For this review, take the finished solid that the model builds, in its own axes (mm). A direction names the side the tool comes from. Give positions to 0.01 mm unless a question says otherwise; leave off trailing zeros. Order: outer loops, then holes, each group sorted by start corner. A loop starts at its lowest first (then second) coordinate and runs counter-clockwise, first axis right, second up. Notation, with made-up numbers: (43.5, 28) - (58.5, 28) arc R30 cw to (58.5, 58) - close; hole circle Ø3 at (45.5, 65.5). An arc over 180 degrees is marked (long way). One line per item, written item: value.
```python
from build123d import *

# Parameters (mm, degrees)
BOSS_EXTRUDE1_DEPTH = 6.35


with BuildPart() as part:
    # Sketch1 → Boss-Extrude1 (new body)
    with BuildSketch(Plane(origin=(0, 0, 0), x_dir=(0, 0, -1), z_dir=(1, 0, 0))):
        Polygon((0, 14.9225), (0, 6.35), (0, 0), (6.35, 0), (18.7325, 0), (18.7325, 6.35), (35.8775, 6.35), (35.8775, 0), (53.0225, 0), (53.0225, 6.35), (70.1675, 6.35), (70.1675, 0), (82.55, 0), (88.9, 0), (88.9, 6.35), (88.9, 14.9225), (82.55, 14.9225), (82.55, 32.0675), (88.9, 32.0675), (88.9, 49.2125), (82.55, 49.2125), (82.55, 66.3575), (88.9, 66.3575), (88.9, 83.5025), (82.55, 83.5025), (82.55, 100.6475), (88.9, 100.6475), (88.9, 117.7925), (82.55, 117.7925), (82.55, 134.9375), (88.9, 134.9375), (88.9, 152.0825), (82.55, 152.0825), (82.55, 169.2275), (88.9, 169.2275), (88.9, 186.3725), (82.55, 186.3725), (82.55, 203.5175), (88.9, 203.5175), (88.9, 220.6625), (82.55, 220.6625), (82.55, 237.8075), (88.9, 237.8075), (88.9, 254.9525), (82.55, 254.9525), (82.55, 272.0975), (88.9, 272.0975), (88.9, 289.2425), (82.55, 289.2425), (82.55, 306.3875), (88.9, 306.3875), (88.9, 323.5325), (82.55, 323.5325), (82.55, 340.6775), (88.9, 340.6775), (88.9, 349.25), (70.1675, 349.25), (70.1675, 355.6), (53.0225, 355.6), (53.0225, 349.25), (35.8775, 349.25), (35.8775, 355.6), (18.7325, 355.6), (18.7325, 349.25), (6.35, 349.25), (0, 349.25), (0, 340.6775), (6.35, 340.6775), (6.35, 334.518000001), (6.35, 329.692000001), (6.35, 323.5325), (0, 323.5325), (0, 306.3875), (6.35, 306.3875), (6.35, 289.2425), (0, 289.2425), (0, 272.0975), (6.35, 272.0975), (6.35, 254.9525), (0, 254.9525), (0, 237.8075), (6.35, 237.8075), (6.35, 220.6625), (0, 220.6625), (0, 203.5175), (6.35, 203.5175), (6.35, 186.3725), (0, 186.3725), (0, 169.2275), (6.35, 169.2275), (6.35, 152.0825), (0, 152.0825), (0, 134.9375), (6.35, 134.9375), (6.35, 117.7925), (0, 117.7925), (0, 100.6475), (6.35, 100.6475), (6.35, 83.5025), (0, 83.5025), (0, 66.3575), (6.35, 66.3575), (6.35, 49.2125), (0, 49.2125), (0, 32.0675), (6.35, 32.0675), (6.35, 25.907999999), (6.35, 21.081999999), (6.35, 14.9225), align=None)
    extrude(amount=BOSS_EXTRUDE1_DEPTH)


solid = part.part
```
(1) For P1, Ø3, axis at x = 2, z = -2.5, coming from the +Y side; P2, Ø1.9, axis at x = 3, y = 233, coming from the -Z side; P3, Ø3, axis at x = 4.5, y = 353, coming from the +Z side, all flat-tipped, find the tip position at first contact; note any pin that passes through.
Answers below:
P1: stops at y = 349.25
P2: stops at z = -82.55
P3: stops at z = -18.73
(2) Draft analysis for pull direction Y (two halves, no side actions). For faces 5 (the face through (3, 58, -82.55)), 6 (the face through (3, 0, -9)), 7 (the face through (3, 349.25, -9)), state which applies: pulls with the +Y half, pulls with the -Y half, needs draft (parallel to the pull), parting line crosses it, or undercut.
Answers below:
face 5: undercut
face 6: pulls with the -Y half
face 7: pulls with the +Y half
(3) Machinability: for faces 1 (the face through (3, 3, -35.878)), 2 (the face through (3, 41, -88.9)), 3 (the face through (3, 83.502, -3)), 4 (the face through (3, 332, -82.55)), which of the approach directions +Z, -Z, +X, -X, +Y, -Y give a long, thin tool a straight path to every point of the face, cutting with its end or side? Answer none if there is none.
Answers below:
face 1: +X, -X, -Y
face 2: -Z, +X, -X, +Y, -Y
face 3: +Z, +X, -X
face 4: -Z, +X, -X
(4) Take a section at B-B (y = 130). Write out the cut boundary in (x, z).
Answers below:
outline: (0, -82.55) - (6.35, -82.55) - (6.35, -6.35) - (0, -6.35) - close
(5) Take a section at A-A (z = -46.5). Write out the cut boundary in (x, y), then the cut area to 3 significant figures.
Answers below:
outline: (0, 0) - (6.35, 0) - (6.35, 349.25) - (0, 349.25) - close
area: 2,220 mm^2
(6) Wall thickness on line 1 (Y direction, x = 5.5, z = -7); line 2 (Y direction, x = 2.75, z = -32.5); line 3 (Z direction, x = 5.75, y = 325.5): over which ranges is each line inside the solid? List them lowest first. Write a range as from..to.
Answers below:
line 1: y = 0..349.25
line 2: y = 6.35..355.6
line 3: z = -82.55..-6.35
